Geometry: final body of the model. Coordinates: model frame, mm. A direction names the side the tool comes from. Coordinates: 2 decimals unless noted, no trailing zeros. Write each loop counter-clockwise with the first axis right and the second up, starting at its lowest first coordinate (ties: lowest second). Pieces come first, ordered by that corner, then holes. Notation, with made-up numbers: (-23.75, -28) - (15.25, -28) arc R24 ccw to (15.25, 7) - close; hole circle Ø5 at (62, 70). An arc over 180 degrees is marked (long way). Answer as a JSON object with one key per item and string values. Group by question number.
Item 1: Section D-D on z = -16. Return loops of the section in (x, y).
Item 2: Section A-A on y = 41. Return loops of the section in (x, z), and give its area (3 significant figures).
Item 3: Line query: line 1 along Z through (x, y) = (30, 32); line 2 along Z through (x, y) = (43, -28.5); line 3 along Y through (x, z) = (-12, -17). Output: solid intervals per line, ascending. Write a range as from..to.
Item 4: Mould query, pull axis Y, two halves, no side actions, for faces 1 (the flat face through (23, 40, -14)), 2 (the flat face through (17, 26, -25.5)), 3 (the cylindrical face through (-82.056, 51.138, -30.902)). Classes: pulls with the +Y half, pulls with the -Y half, needs draft (parallel to the pull), parting line crosses it, or undercut.
Item 5: First-contact query: pin 1 Ø12 at (y, z) = (26, -45) entering from -X; pin 2 Ø9 at (x, y) = (-75.5, 47.5) entering from -Z; pin 3 Ø8 at (x, y) = (-35.5, 50.5) entering from -Z. Flat tips, straight axial feed; report the tip coordinate or a pass-through.
Item 6: Section C-C on z = -28. Return loops of the section in (x, y) (1 decimal).
Item 7: Section B-B on x = -71. Return loops of the section in (y, z).
Item 8: Set-up query: faces 4 (the flat face through (-29, 51, -31)), 5 (the flat face through (-5, -22, -2)), 6 (the flat face through (-15, -26, -60)), 7 (the flat face through (60, -36, -38)). Return all of +Z, -Z, +X, -X, +Y, -Y with unobstructed straight access to the full face (end or side cutting, diameter ignored); none if empty.
```python
from build123d import *

# Parameters (mm, degrees)
BOSS_EXTRUDE1_DEPTH = 65
BOSS_EXTRUDE2_START = -11
SKETCH1_4_R         = 18.5
SKETCH1_4_R_2       = 11
BOSS_EXTRUDE2_DEPTH = 14
BOSS_EXTRUDE3_START = -19
SKETCH1_5_R         = 15
SKETCH1_5_R_2       = 6.355
BOSS_EXTRUDE3_DEPTH = 19
BOSS_EXTRUDE4_START = -24
SKETCH1_6_R         = 15
SKETCH1_6_R_2       = 7.1475
BOSS_EXTRUDE4_DEPTH = 14
BOSS_EXTRUDE5_START = -25.5
BOSS_EXTRUDE5_DEPTH = 11
BOSS_EXTRUDE6_START = -25.5
BOSS_EXTRUDE6_DEPTH = 11
BOSS_EXTRUDE8_START = -14
BOSS_EXTRUDE8_DEPTH = 11
BOSS_EXTRUDE9_START = -5
SKETCH1_11_R        = 3.5
BOSS_EXTRUDE9_DEPTH = 55


with BuildPart() as part:
    # Sketch1 → Boss-Extrude1 (new body)
    with BuildSketch(Plane.XY):
        with BuildLine():
            ThreePointArc((2.423237338, 29.901971855), (1.212609656, 29.975482946), (0, 30))
            Line((0, 30), (-19, 30))
            Line((-19, 30), (-19, 15))
            Line((-19, 15), (0, 15))
            ThreePointArc((0, 15), (15, 0), (0, -15))
            Line((0, -15), (-5, -15))
            Line((-5, -15), (-5, -30))
            Line((-5, -30), (0, -30))
            ThreePointArc((0, -30), (26.089312829, -14.810393516), (25.759532638, 15.376816259))
            ThreePointArc((25.759532638, 15.376816259), (15.852828365, 25.469350852), (2.423237338, 29.901971855))
        make_face()
    extrude(amount=-BOSS_EXTRUDE1_DEPTH)



with BuildPart() as body_2:
    # Sketch1_4 → Boss-Extrude2 (new body)
    with BuildSketch(Plane.XY.offset(BOSS_EXTRUDE2_START)):
        with Locations((27, 70)):
            Circle(SKETCH1_4_R)
        with Locations((27, 70)):
            Circle(SKETCH1_4_R_2, mode=Mode.SUBTRACT)
    extrude(amount=-BOSS_EXTRUDE2_DEPTH)


with BuildPart() as body_3:
    # Sketch1_5 → Boss-Extrude3 (new body)
    with BuildSketch(Plane.XY.offset(BOSS_EXTRUDE3_START)):
        with Locations((54, -33)):
            Circle(SKETCH1_5_R)
        with Locations((54, -33)):
            Circle(SKETCH1_5_R_2, mode=Mode.SUBTRACT)
    extrude(amount=-BOSS_EXTRUDE3_DEPTH)


with BuildPart() as body_4:
    # Sketch1_6 → Boss-Extrude4 (new body)
    with BuildSketch(Plane.XY.offset(BOSS_EXTRUDE4_START)):
        with Locations((-71, 41)):
            Circle(SKETCH1_6_R)
        with Locations((-71, 41)):
            Circle(SKETCH1_6_R_2, mode=Mode.SUBTRACT)
    extrude(amount=-BOSS_EXTRUDE4_DEPTH)


with BuildPart() as part_1:
    add(part.part)

    add(body_4.part)  # Boss-Extrude5 merges body 4
    # Sketch1_7 → Boss-Extrude5 (add)
    with BuildSketch(Plane.XY.offset(BOSS_EXTRUDE5_START)):
        with BuildLine():
            Line((-19, 30), (0, 30))
            ThreePointArc((0, 30), (1.212609656, 29.975482946), (2.423237338, 29.901971855))
            Line((2.423237338, 29.901971855), (10.166256776, 49.976466693))
            ThreePointArc((10.166256776, 49.976466693), (5.10882563, 50.743471508), (0, 51))
            Line((0, 51), (-59.819660113, 51))
            ThreePointArc((-59.819660113, 51), (-56.987414616, 46.352331347), (-56, 41))
            ThreePointArc((-56, 41), (-62.175451499, 28.870393916), (-75.616979166, 26.728227041))
            Line((-75.616979166, 26.728227041), (-44, 16.5))
            Line((-44, 16.5), (-44, 15))
            Line((-44, 15), (-19, 15))
            Line((-19, 15), (-19, 30))
        make_face()
    extrude(amount=-BOSS_EXTRUDE5_DEPTH)


    add(body_3.part)  # Boss-Extrude6 merges body 3
    # Sketch1_8 → Boss-Extrude6 (add)
    with BuildSketch(Plane.XY.offset(BOSS_EXTRUDE6_START)):
        with BuildLine():
            Line((34.363921616, 37.684491388), (25.759532638, 15.376816259))
            ThreePointArc((25.759532638, 15.376816259), (26.089312829, -14.810393516), (0, -30))
            Line((0, -30), (22.250984267, -30))
            ThreePointArc((22.250984267, -30), (33.101317429, -32.861811207), (41.128777406, -40.702702703))
            ThreePointArc((41.128777406, -40.702702703), (47.097213206, -19.682660383), (67.713804516, -26.922865338))
            Line((67.713804516, -26.922865338), (46.626935354, 20.662257852))
            ThreePointArc((46.626935354, 20.662257852), (41.380174442, 29.81075583), (34.363921616, 37.684491388))
        make_face()
        with BuildLine():
            Line((10.166256776, 49.976466693), (2.423237338, 29.901971855))
            ThreePointArc((2.423237338, 29.901971855), (15.852828365, 25.469350852), (25.759532638, 15.376816259))
            Line((25.759532638, 15.376816259), (34.363921616, 37.684491388))
            ThreePointArc((34.363921616, 37.684491388), (23.097778273, 45.469689232), (10.166256776, 49.976466693))
        make_face()
    extrude(amount=-BOSS_EXTRUDE6_DEPTH)


    add(body_2.part)  # Boss-Extrude8 merges body 2
    # Sketch1_9 → Boss-Extrude8 (add)
    with BuildSketch(Plane.XY.offset(BOSS_EXTRUDE8_START)):
        with BuildLine():
            Line((10.166256776, 49.976466693), (2.423237338, 29.901971855))
            ThreePointArc((2.423237338, 29.901971855), (15.852828365, 25.469350852), (25.759532638, 15.376816259))
            Line((25.759532638, 15.376816259), (34.363921616, 37.684491388))
            ThreePointArc((34.363921616, 37.684491388), (23.097778273, 45.469689232), (10.166256776, 49.976466693))
        make_face()
        with BuildLine():
            Line((13.156184416, 57.728130946), (10.166256776, 49.976466693))
            ThreePointArc((10.166256776, 49.976466693), (23.097778273, 45.469689232), (34.363921616, 37.684491388))
            Line((34.363921616, 37.684491388), (44.26053068, 63.342366738))
            ThreePointArc((44.26053068, 63.342366738), (30.286091355, 51.794187642), (13.156184416, 57.728130946))
        make_face()
    extrude(amount=-BOSS_EXTRUDE8_DEPTH)

    # Sketch1_11 → Boss-Extrude9 (add)
    with BuildSketch(Plane.XY.offset(BOSS_EXTRUDE9_START)):
        with BuildLine():
            Line((-19, -30), (-5, -30))
            Line((-5, -30), (-5, -15))
            Line((-5, -15), (-20.839490527, -15))
            ThreePointArc((-20.839490527, -15), (-24, -23.000372662), (-19, -30))
        make_face()
        with Locations((-15.066920643, -21.904885006)):
            Circle(SKETCH1_11_R, mode=Mode.SUBTRACT)
    extrude(amount=-BOSS_EXTRUDE9_DEPTH)


solid = part_1.part
```
Checks:
{
 "1": {"outline": "(-20.84, -15) arc R9 ccw to (-19, -30) - (0, -30) arc R30 ccw to (25.76, 15.38) - (44.26, 63.34) arc R18.5 ccw (long way) to (13.16, 57.73) - (2.42, 29.9) arc R30 ccw to (0, 30) - (-19, 30) - (-19, 15) - (0, 15) arc R15 cw to (0, -15) - close; hole circle Ø7 at (-15.07, -21.9); hole circle Ø22 at (27, 70)"},
 "2": {"outline": "(-86, -38) - (-78.15, -38) - (-78.15, -24) - (-86, -24) - close; (-63.85, -38) - (-56, -38) - (-56, -36.5) - (30.33, -36.5) - (30.33, -25.5) - (-56, -25.5) - (-56, -24) - (-63.85, -24) - close; (6.7, -25) - (35.64, -25) - (35.64, -14) - (6.7, -14) - close", "area": "1,490 mm^2"},
 "3": {"line 1": "-36.5..-25.5, -25..-14", "line 2": "-38..-19", "line 3": "-30..-23.59, -20.22..-15, 15..30"},
 "4": {"face 1": "undercut", "face 2": "needs draft", "face 3": "parting line crosses it"},
 "5": {"pin 1": "x = -19", "pin 2": "z = -38", "pin 3": "z = -36.5"},
 "6": {"outline": "(-75.6, 26.7) - (-44, 16.5) - (-44, 15) - (0, 15) arc R15 cw to (0, -15) - (-20.8, -15) arc R9 ccw to (-19, -30) - (22.3, -30) arc R22 cw to (41.1, -40.7) arc R15 ccw to (67.7, -26.9) - (46.6, 20.7) arc R51 ccw to (0, 51) - (-59.8, 51) arc R15 ccw (long way) to start; hole circle Ø14.3 at (-71, 41); hole circle Ø7 at (-15.1, -21.9); hole circle Ø12.7 at (54, -33)"},
 "7": {"outline": "(25.23, -36.5) - (26, -36.5) - (26, -38) - (33.85, -38) - (33.85, -24) - (26, -24) - (26, -25.5) - (25.23, -25.5) - close; (48.15, -38) - (56, -38) - (56, -24) - (48.15, -24) - close"},
 "8": {"face 4": "+Z, -Z, +X, +Y", "face 5": "+Z, -X, -Y", "face 6": "-Z, -X, -Y", "face 7": "-Z, +X, +Y, -Y"}
}
